For this review, take the finished solid that the model builds, in its own axes (mm). A direction names the side the tool comes from. Give positions to 0.01 mm unless a question says otherwise; leave off trailing zeros. Loops run counter-clockwise (first coordinate to the right, second up) from the corner with the lowest first, then second, coordinate; pieces in that order, holes last. Notation, with made-up numbers: (-7.5, -10.5) - (39.5, -10.5) arc R12 ccw to (39.5, 0.5) - close; hole circle Ø5 at (-1.5, -1.5). An arc over 180 degrees is marked (long way). Answer as CSV lines item,"result".
from build123d import *

# Parameters (mm, degrees)
SKETCH_1_W                 = 146
SKETCH_1_H                 = 48
EXTRUDE_146X48_DEPTH       = 3
CUT_EXTRUDE_492_DEPTH      = 80.76214641
CUT_EXTRUDE_492_DEPTH_BACK = 80.76214641
SKETCH_2_W                 = 40
SKETCH_2_H                 = 36
F_6MM_START                = -6
SKETCH_3_R                 = 2.7
F_6MM_DEPTH                = 6
F_2P8_3P4_DEPTH            = 80.931220434
F_2P8_3P4_DEPTH_BACK       = 80.931220434
SKETCH_4_R                 = 1.4
SKETCH_4_R_2               = 1.7


with BuildPart() as part:
    # 草图1 → 相机横梁146x48 (new body)
    with BuildSketch(Plane.XY):
        with Locations((0, -8)):
            Rectangle(SKETCH_1_W, SKETCH_1_H)
    extrude(amount=EXTRUDE_146X48_DEPTH)

    # 草图2 → Cut-Extrude 492 (cut, two sides: drawn at the far end of the back side and taken through both)
    with BuildSketch(Plane.XY.offset(-CUT_EXTRUDE_492_DEPTH_BACK)):
        with Locations((-38, -8)):
            Rectangle(SKETCH_2_W, SKETCH_2_H)
        with Locations((38, -8)):
            Rectangle(SKETCH_2_W, SKETCH_2_H)
    extrude(amount=CUT_EXTRUDE_492_DEPTH + CUT_EXTRUDE_492_DEPTH_BACK, mode=Mode.SUBTRACT)

    # 草图3 → 背面6mm间隔柱 (add)
    with BuildSketch(Plane.XY.offset(F_6MM_START)):
        with Locations((-10.5, -6.75)):
            Circle(SKETCH_3_R)
        with Locations((-10.5, 6.75)):
            Circle(SKETCH_3_R)
        with Locations((10.5, -6.75)):
            Circle(SKETCH_3_R)
        with Locations((10.5, 6.75)):
            Circle(SKETCH_3_R)
    extrude(amount=F_6MM_DEPTH)

    # 草图4 → 相机2p8孔与梁端3p4孔 (cut, two sides: drawn at the far end of the back side and taken through both)
    with BuildSketch(Plane.XY.offset(-F_2P8_3P4_DEPTH_BACK)):
        with Locations((-10.5, -6.75)):
            Circle(SKETCH_4_R)
        with Locations((-10.5, 6.75)):
            Circle(SKETCH_4_R)
        with Locations((10.5, -6.75)):
            Circle(SKETCH_4_R)
        with Locations((10.5, 6.75)):
            Circle(SKETCH_4_R)
        with Locations((-66.6, -25)):
            Circle(SKETCH_4_R_2)
        with Locations((66.6, -25)):
            Circle(SKETCH_4_R_2)
    extrude(amount=F_2P8_3P4_DEPTH + F_2P8_3P4_DEPTH_BACK, mode=Mode.SUBTRACT)


solid = part.part
1) Consider section D-D on y = -6.75. Write out the cut boundary in (x, z), and give its area (3 significant figures).
From the geometry:
outline,"(-73, 0) - (-58, 0) - (-58, 3) - (-73, 3) - close; (-18, 0) - (-13.2, 0) - (-13.2, -6) - (-11.9, -6) - (-11.9, 3) - (-18, 3) - close; (-9.1, -6) - (-7.8, -6) - (-7.8, 0) - (7.8, 0) - (7.8, -6) - (9.1, -6) - (9.1, 3) - (-9.1, 3) - close; (11.9, -6) - (13.2, -6) - (13.2, 0) - (18, 0) - (18, 3) - (11.9, 3) - close; (58, 0) - (73, 0) - (73, 3) - (58, 3) - close"
area,"212 mm^2"
2) Wall thickness on line 1 (X direction, y = -13.5, z = 1.5); line 2 (Y direction, x = 10.5, z = -2.25); line 3 (X direction, y = -25, z = 1.15): over which ranges is each line inside the solid? List them lowest first. Write a range as from..to.
From the geometry:
line 1,"x = -73..-58, -18..18, 58..73"
line 2,"y = -9.45..-8.15, -5.35..-4.05, 4.05..5.35, 8.15..9.45"
line 3,"x = -73..-68.3, -64.9..-58, -18..18, 58..64.9, 68.3..73"
3) Insertion check: P1, Ø2, axis at x = -29.5, z = -1.5, coming from the +Y side; P2, Ø3, axis at y = -4.5, z = -4, coming from the -X side; P3, Ø1, axis at y = 4, z = -3, coming from the -X side; P4, Ø14.5, axis at x = 0.5, y = -10, coming from the -Z side. Each pin has a flat end and moves straight along its axis. Give the tip position at first contact, or say it passes through.
From the geometry:
P1,"passes through"
P2,"stops at x = -13.09"
P3,"stops at x = -11.99"
P4,"stops at z = 0"
4) Draft analysis for pull direction Y (two halves, no side actions). For faces 3 (the cylindrical face through (-9.254, 4.355, -3.042)), 4 (the flat face through (12, 6, -6)), 5 (the flat face through (-1, -32, 1)), state which applies: pulls with the +Y half, pulls with the -Y half, needs draft (parallel to the pull), parting line crosses it, or undercut.
From the geometry:
face 3,"undercut"
face 4,"needs draft"
face 5,"pulls with the -Y half"
5) Machinability: for faces 1 (the flat face through (-9, -8, -6)), 2 (the flat face through (18, -8, 1)), which of the approach directions +Z, -Z, +X, -X, +Y, -Y give a long, thin tool a straight path to every point of the face, cutting with its end or side? Answer none if there is none.
From the geometry:
face 1,"-Z, +X, -X, +Y, -Y"
face 2,"+Z, -Z"
6) Consider section A-A on z = -3.5. Write out the cut boundary in (x, y), and give its area (3 significant figures).
From the geometry:
outline,"circle Ø5.4 at (-10.5, -6.75); circle Ø5.4 at (-10.5, 6.75); circle Ø5.4 at (10.5, -6.75); circle Ø5.4 at (10.5, 6.75); hole circle Ø2.8 at (-10.5, -6.75); hole circle Ø2.8 at (-10.5, 6.75); hole circle Ø2.8 at (10.5, -6.75); hole circle Ø2.8 at (10.5, 6.75)"
area,"67.0 mm^2"
7) Consider section C-C on x = 10.5. Write out the cut boundary in (y, z), and give its area (3 significant figures).
From the geometry:
outline,"(-32, 0) - (-9.45, 0) - (-9.45, -6) - (-8.15, -6) - (-8.15, 3) - (-32, 3) - close; (-5.35, -6) - (-4.05, -6) - (-4.05, 0) - (4.05, 0) - (4.05, -6) - (5.35, -6) - (5.35, 3) - (-5.35, 3) - close; (8.15, -6) - (9.45, -6) - (9.45, 0) - (16, 0) - (16, 3) - (8.15, 3) - close"
area,"158 mm^2"
8) Consider section B-B on y = -19.5. Write out the cut boundary in (x, z).
From the geometry:
outline,"(-73, 0) - (-58, 0) - (-58, 3) - (-73, 3) - close; (-18, 0) - (18, 0) - (18, 3) - (-18, 3) - close; (58, 0) - (73, 0) - (73, 3) - (58, 3) - close"
